Can you work these out from the model? Positions are in its coordinate system, mm. A direction names the side the tool comes from. Give positions to 0.01 mm unless a question says otherwise; leave off trailing zeros. Order: outer loops, then holes, each group sorted by start corner. A loop starts at its lowest first (then second) coordinate and runs counter-clockwise, first axis right, second up. Notation, with made-up numbers: (-40, 62.25) - (13, 62.25) arc R29 ccw to (13, 99.25) - close; hole circle Ø4 at (80.5, 64). An arc over 180 degrees is marked (long way). Answer as a JSON object with one key per item and string values.
```python
from build123d import *

# Parameters (mm, degrees)
F2_R     = 19.05
F3_DEPTH = 25.4


with BuildPart() as f1:
    # F0 (on Front) → F1 (revolve)
    with BuildSketch(Plane.XZ):
        with BuildLine():
            Line((-38.1, 0), (0, 0))
            Line((0, 0), (0, 101.6))
            Line((0, 101.6), (-38.1, 101.6))
            Line((-38.1, 101.6), (-38.1, 94.693672))
            ThreePointArc((-38.1, 94.693672), (-31.75, 88.343672), (-38.1, 81.993672))
            Line((-38.1, 81.993672), (-38.1, 26.956592))
            ThreePointArc((-38.1, 26.956592), (-31.75, 20.606592), (-38.1, 14.256592))
            Line((-38.1, 14.256592), (-38.1, 0))
        make_face()
    revolve(axis=Axis((0, 0, 50.8), (0, 0, 1)))

    # F2 (on Front) → F3 (cut)
    with BuildSketch(Plane.XZ):
        with Locations((0, 53.649068)):
            Circle(F2_R)
    extrude(amount=-F3_DEPTH, mode=Mode.SUBTRACT)


solid = f1.part
```
Q1. If we section it at C-C, the plane y = 33: Count the separate pieces of the cut face and the enclosed holes in it, then the cut area to 3 significant figures.
Recorded:
{"separate pieces": "3", "enclosed holes": "0", "area": "3,090 mm^2"}
Q2. If we section it at A-A, the plane x = 0: Please give me the cut outline in (y, z).
Recorded:
{"outline": "(-38.1, 0) - (38.1, 0) - (38.1, 14.26) arc R6.35 cw to (38.1, 26.96) - (38.1, 81.99) arc R6.35 cw to (38.1, 94.69) - (38.1, 101.6) - (-38.1, 101.6) - (-38.1, 94.69) arc R6.35 cw to (-38.1, 81.99) - (-38.1, 26.96) arc R6.35 cw to (-38.1, 14.26) - close; hole (0, 34.6) - (25.4, 34.6) - (25.4, 72.7) - (0, 72.7) - close"}
Q3. I'm going to push flat-ended pins straight in: pin 1 Ø6 at (y, z) = (13, 43.5) entering from +X; pin 2 Ø6 at (y, z) = (-25.5, 48) entering from +X; pin 3 Ø10 at (x, z) = (-14.5, 18) entering from -Y; pin 4 Ø8 at (x, y) = (-14, 14) entering from -Z. Where does each tip first touch, or does it pass through?
Recorded:
{"pin 1": "stops at x = 36.76", "pin 2": "stops at x = 30.75", "pin 3": "stops at y = -36.42", "pin 4": "stops at z = 0"}
Q4. I need wall thicknesses on L1, parallel to Z at x = 17, y = 33.5; L2, parallel to Z at x = 20.5, y = -30.5; L3, parallel to Y at x = 0.5, z = 55. Which ranges of each line are inside material? Lowest first, please.
Recorded:
{"L1": "z = 0 to 14.28, 26.93 to 82.02, 94.67 to 101.6", "L2": "z = 0 to 14.4, 26.81 to 82.14, 94.55 to 101.6", "L3": "y = -38.1 to 0, 25.4 to 38.1"}
Q5. If we section it at D-D, the plane z = 48.5: Please give me the cut outline in (x, y).
Recorded:
{"outline": "circle Ø76.2 at (0, 0); hole (-18.34, 0) - (18.34, 0) - (18.34, 25.4) - (-18.34, 25.4) - close"}
Q6. If we section it at B-B, the plane z = 32: Please give me the cut outline in (x, y), then the cut area to 3 significant figures.
Recorded:
{"outline": "circle Ø76.2 at (0, 0)", "area": "4,560 mm^2"}
Q7. Which directions (+Z, -Z, +X, -X, +Y, -Y) give clear straight access to the entire face, cutting with the end or side of a thin tool? Please do faces 1 (the face through (0, 25.4, 54)), 2 (the face through (1, -1, 0)).
Recorded:
{"face 1": "none", "face 2": "-Z, +X, -X, +Y, -Y"}
Q8. We'd pull the mould along X, two halves only. Please class faces 3 (the face through (0, 0, 54)), 4 (the face through (30.235, 23.183, 7.028)), 5 (the face through (-1, -1, 101.6)): released by +X, released by -X, zero draft, split by the parting line, or undercut.
Recorded:
{"face 3": "undercut", "face 4": "split by the parting line", "face 5": "zero draft"}
